CAD build for the part. Positions are in the model's coordinates, mm. A direction names the side the tool comes from. Coordinates: 2 decimals unless noted, no trailing zeros. Write each loop counter-clockwise with the first axis right and the second up, starting at its lowest first coordinate (ties: lowest second). Pieces come first, ordered by that corner, then holes. Notation, with made-up numbers: M 83.5,46 L 121.5,46 A10 ccw 121.5,51 Z; hole C 25,34.5 d3. An arc over 180 degrees is marked long. Answer as CSV lines item,"result". Start each with the question number.
```python
from build123d import *

# Parameters (mm, degrees)
F2_DEPTH = 3
F1_W     = 10.2
F1_H     = 6.1991158426
F1_H_2   = 23.2707020342
F3_DEPTH = 3


with BuildPart() as f2:
    # F0 (on Top) → F2 (new body)
    with BuildSketch(Plane.XY):
        with BuildLine():
            ThreePointArc((11.3067825639, 29.4007936636), (11.4515937375, 30.4459601281), (11.4999999642, 31.5))
            ThreePointArc((11.4999999642, 31.5), (-1.0540399207, 42.9515937721), (-11.3067826307, 29.4007936379))
            ThreePointArc((-11.3067826307, 29.4007936379), (-3.58e-08, 31.5), (11.3067825639, 29.4007936636))
        make_face()
        with BuildLine():
            ThreePointArc((11.3067825639, 29.4007936636), (-3.58e-08, 31.5), (-11.3067826307, 29.4007936379))
            ThreePointArc((-11.3067826307, 29.4007936379), (-2.27e-08, 20), (11.3067825639, 29.4007936636))
        make_face()
        with BuildLine():
            ThreePointArc((11.3067825639, 29.4007936636), (-2.27e-08, 20), (-11.3067826307, 29.4007936379))
            ThreePointArc((-11.3067826307, 29.4007936379), (-27.2798002371, 15.749999969), (-31.1152254861, -4.9084358964))
            ThreePointArc((-31.1152254861, -4.9084358964), (-20.641178009, -6.3596488455), (-15.7798002013, -15.750000031))
            ThreePointArc((-15.7798002013, -15.750000031), (-16.8354091384, -20.5629716001), (-19.8084428665, -24.4923578123))
            ThreePointArc((-19.8084428665, -24.4923578123), (3.58e-08, -31.5), (19.8084429222, -24.4923577673))
            ThreePointArc((19.8084429222, -24.4923577673), (17.320508087, -9.9999999803), (31.1152254973, -4.9084358257))
            ThreePointArc((31.1152254973, -4.9084358257), (31.4036590477, -2.4617470256), (31.5, 0))
            ThreePointArc((31.5, 0), (25.965492974, 17.8337650152), (11.3067825639, 29.4007936636))
        make_face()
        with BuildLine():
            ThreePointArc((-19.8084428665, -24.4923578123), (-27.2798002013, -15.750000031), (-31.1152254861, -4.9084358964))
            ThreePointArc((-31.1152254861, -4.9084358964), (-37.2390923383, -21.5000000423), (-19.8084428665, -24.4923578123))
        make_face()
        with BuildLine():
            ThreePointArc((-15.7798002013, -15.750000031), (-20.641178009, -6.3596488455), (-31.1152254861, -4.9084358964))
            ThreePointArc((-31.1152254861, -4.9084358964), (-27.2798002013, -15.750000031), (-19.8084428665, -24.4923578123))
            ThreePointArc((-19.8084428665, -24.4923578123), (-16.8354091384, -20.5629716001), (-15.7798002013, -15.750000031))
        make_face()
        with BuildLine():
            ThreePointArc((19.8084429222, -24.4923577673), (27.2798002371, -15.749999969), (31.1152254973, -4.9084358257))
            ThreePointArc((31.1152254973, -4.9084358257), (17.320508087, -9.9999999803), (19.8084429222, -24.4923577673))
        make_face()
        with BuildLine():
            ThreePointArc((38.7798002371, -15.749999969), (36.6701514151, -9.111377766), (31.1152254973, -4.9084358257))
            ThreePointArc((31.1152254973, -4.9084358257), (27.2798002371, -15.749999969), (19.8084429222, -24.4923577673))
            ThreePointArc((19.8084429222, -24.4923577673), (32.0927718181, -26.1943910265), (38.7798002371, -15.749999969))
        make_face()
    extrude(amount=F2_DEPTH)

    # F1 (on Top) → F3 (cut)
    with BuildSketch(Plane.XY):
        with BuildLine():
            Line((5.1, 23), (5.1, 16.8008841574))
            Line((5.1, 16.8008841574), (-5.1, 16.8008841574))
            Line((-5.1, 16.8008841574), (-5.1, 23))
            Line((-5.1, 23), (-8, 23))
            ThreePointArc((-8, 23), (-18.6066017178, 18.6066017178), (-23, 8))
            Line((-23, 8), (-23, -8))
            ThreePointArc((-23, -8), (-18.6066017178, -18.6066017178), (-8, -23))
            Line((-8, -23), (8, -23))
            ThreePointArc((8, -23), (18.6066017178, -18.6066017178), (23, -8))
            Line((23, -8), (23, 8))
            ThreePointArc((23, 8), (18.6066017178, 18.6066017178), (8, 23))
            Line((8, 23), (5.1, 23))
        make_face()
        with Locations((0, 19.9004420787)):
            Rectangle(F1_W, F1_H)
        with Locations((0, 34.6353510171)):
            Rectangle(F1_W, F1_H_2)
    extrude(amount=F3_DEPTH, mode=Mode.SUBTRACT)


solid = f2.part
```
1) Pin check, flat tips, straight feed: P1, Ø1, axis at x = -3, z = 1, coming from the -Y side; P2, Ø1.5, axis at y = 29.5, z = 2, coming from the -X side; P3, Ø0.9, axis at x = 6.5, z = 2, coming from the -Y side. Stop position of each tip, or through.
2) Band-saw the part on D-D, the plane x = 25. List the corners of the cut face in (y, z), plus the area to 3 significant figures.
3) Band-saw the part on C-C, the plane z = 2.05. List the corners of the cut face in (x, y).
4) Two-plate mould, pull along Y, no slides. Class faces 4 (the cylindrical face through (-0.3, -31.5, 1.5)), 5 (the cylindrical face through (-18.49, 18.72, 1.48)), 6 (the flat face through (-5.1, 32, 1)), 7 (the cylindrical face through (18.49, -18.72, 1.48)): pulls with the +Y half, pulls with the -Y half, needs draft (parallel to the pull), parting line crosses it, or undercut.
5) Band-saw the part on A-A, the plane x = -22. List the corners of the cut face in (y, z), plus the area to 3 significant figures.
6) Tool access for faces 1 (the flat face through (3, -25, 3)), 2 (the flat face through (0, -23, 1)), 3 (the flat face through (5.1, 32, 1)): list every direction of +Z, -Z, +X, -X, +Y, -Y with a clear straight run to the whole face (end or side of a thin tool).
7) Probe L1, parallel to Y at x = 1, z = 1.3; L2, parallel to X at y = 18, z = 2; L3, parallel to X at y = -21, z = 0.45. List the from-to ranges inside material, lowest first. Write a range as [from, to].
8) Band-saw the part on B-B, the plane y = 19. List the corners of the cut face in (x, z).
Result sheet:
1,P1,"stops at y = -31.4"
1,P2,"stops at x = -12.87"
1,P3,"stops at y = -30.91"
2,outline,"M -27.02,0 L 19.16,0 L 19.16,3 L -27.02,3 Z"
2,area,"139 mm²"
3,outline,"M -31.12,-4.91 A11.5 ccw long -19.81,-24.49 A31.5 ccw 19.81,-24.49 A11.5 ccw long 31.12,-4.91 A31.5 ccw 11.31,29.4 A11.5 ccw 5.1,41.81 L 5.1,23 L 8,23 A15 cw 23,8 L 23,-8 A15 cw 8,-23 L -8,-23 A15 cw -23,-8 L -23,8 A15 cw -8,23 L -5.1,23 L -5.1,41.81 A11.5 ccw -11.31,29.4 A31.5 ccw Z"
4,face 4,"pulls with the -Y half"
4,face 5,"undercut"
4,face 6,"needs draft"
4,face 7,"undercut"
5,outline,"M -25.97,0 L -13.39,0 L -13.39,3 L -25.97,3 Z; M 13.39,0 L 22.54,0 L 22.54,3 L 13.39,3 Z"
5,area,"65.2 mm²"
6,face 1,"+Z, +X, -X, +Y, -Y"
6,face 2,"+Z, -Z"
6,face 3,"+Z, -Z, +Y"
7,L1,"y = [-31.48, -23]"
7,L2,"x = [-25.85, -19.18], [19.18, 25.85]"
7,L3,"x = [-37.51, -15.48], [15.48, 37.51]"
8,outline,"M -25.12,0 L -18.2,0 L -18.2,3 L -25.12,3 Z; M 18.2,0 L 25.12,0 L 25.12,3 L 18.2,3 Z"
